from build123d import *

# Parameters (mm, degrees)
EXTRUDE_1_DEPTH       = 7
FILLET_1_R            = 10
CHAMFER_1_SIZE        = 5
CHAMFER_2_SIZE        = 2
SKETCH_3_R            = 4
CUT_EXTRUDE_2_DEPTH   = 98.811761039
SKETCH_5_W            = 7.308921848
SKETCH_5_H            = 35.296607786
CUT_EXTRUDE_2_2_DEPTH = 98.534926302


with BuildPart() as part:
    # Эскиз1 → Вытянуть1 (new body)
    with BuildSketch(Plane(origin=(0, 0, 0), x_dir=(0, 0, -1), z_dir=(1, 0, 0))):
        Polygon((62.822655934, -30.891323454), (59.120013374, -21.327683482), (30.956731402, -21.327683482), (30.956731402, -0.888409733), (92.539330922, -0.888409733), (92.539330922, -30.896809382), align=None)
    extrude(amount=-EXTRUDE_1_DEPTH)

    # Скругление1
    fillet_1_edges = [part.edges().sort_by_distance(p)[0] for p in [
        (-3.5, -21.327683482, -59.120013374),
    ]]
    fillet(fillet_1_edges, radius=FILLET_1_R)

    # Фаска1
    chamfer_1_edges = [part.edges().sort_by_distance(p)[0] for p in [
        (-3.5, -21.327683482, -30.956731402),
        (-3.5, -0.888409733, -30.956731402),
    ]]
    chamfer(chamfer_1_edges, length=CHAMFER_1_SIZE)

    # Фаска2
    chamfer_2_edges = [part.edges().sort_by_distance(p)[0] for p in [
        (0, -15.892609557, -92.539330922),
    ]]
    chamfer(chamfer_2_edges, length=CHAMFER_2_SIZE)

    # Эскиз3 → Cut-Extrude 2 (cut, through all)
    with BuildSketch(Plane.ZY.offset(7)):
        with Locations((-44.770273228, -12.131888622)):
            Circle(SKETCH_3_R)
    extrude(amount=-CUT_EXTRUDE_2_DEPTH, mode=Mode.SUBTRACT)

    # Эскиз5 → Cut-Extrude 2 2 (cut, through all)
    with BuildSketch(Plane(origin=(0, -30.879724855, 0.005700636), x_dir=(1, 0, 0), z_dir=(0, -0.9999999829599957, 0.0001846077143906597))):
        with Locations((-9.634460924, -46.111441198)):
            Rectangle(SKETCH_5_W, SKETCH_5_H)
    extrude(amount=-CUT_EXTRUDE_2_2_DEPTH, mode=Mode.SUBTRACT)


solid = part.part
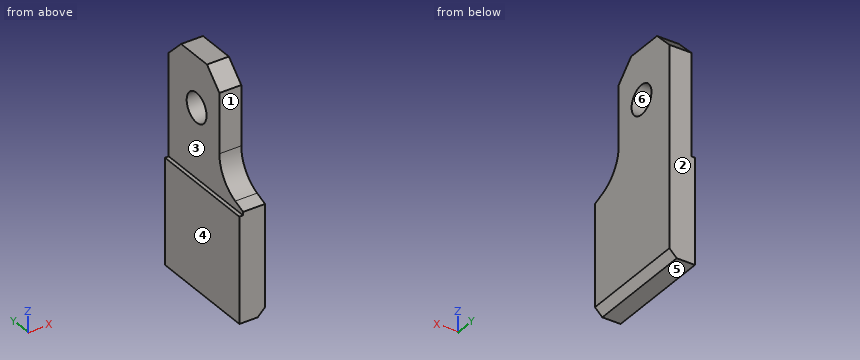
For this review, take the finished solid that the model builds, in its own axes (mm). Face numbers are marked on the shaded views. A direction names the side the tool comes from. Round coordinates to 2 decimals unless told otherwise and drop trailing zeros. Loops run counter-clockwise (first coordinate to the right, second up) from the corner with the lowest first, then second, coordinate; pieces in that order, holes last. Notation, with made-up numbers: (62, 86.5) - (94, 86.5) arc R20 ccw to (94, 94.5) - close; hole circle Ø5 at (63.25, 67.5). An arc over 180 degrees is marked (long way). Put each result on its own line as item: value. Start each with the question number.
1. For the marked faces 1, 2 and 3, list the 3-axis set-ups (+Z, -Z, +X, -X, +Y, -Y) from which the entire face can be reached by the end or side of a thin tool; tool diameter is ignored.
2. Consider section B-B on x = -1. State the section outline as (y, z) points, plus the area to 3 significant figures.
3. Consider section A-A on y = -13.5. State the section outline as (x, z) points, plus the area to 3 significant figures.
4. Consider section C-C on z = -43.5. State the section outline as (x, y) points.
5. Consider section D-D on y = -24.5. State the section outline as (x, z) points, plus the area to 3 significant figures.
6. For probe 1 along X at (y, z) = (-11, -35.5); probe 2 along Y at (x, z) = (-0.25, -80.5); probe 3 along Y at (x, z) = (-2, -40), list the stretches that pass through material, from the lowest coordinate up. Write a range as [from, to].
7. Insertion check: P1, Ø9, axis at y = -18.5, z = -51, coming from the -X side; P2, Ø0.8, axis at x = -6.5, y = -20.5, coming from the +Z side. Each pin has a flat end and moves straight along its axis. Give the tip position at first contact, or say it passes through.
8. Mouldability with a two-part tool opening along Z and no side actions: class the marked faces 4, 5 and 6 as +Z half, -Z half, draft (parallel to the pull), parting line (faces both ways), or undercut.
Result sheet:
1. face 1: +Z, +X, -X, -Y
1. face 2: +Z, -Z, +X, -X, +Y
1. face 3: +Z, -X, +Y, -Y
2. outline: (-30.9, -91.54) - (-0.89, -91.54) - (-0.89, -35.96) - (-5.89, -30.96) - (-16.33, -30.96) - (-21.33, -35.96) - (-21.33, -52.27) arc R10 cw to (-27.72, -61.59) - (-30.89, -62.82) - close; hole circle Ø8 at (-12.13, -44.77)
2. area: 1,460 mm^2
3. outline: (-7, -92.54) - (-2, -92.54) - (0, -90.54) - (0, -48.53) - (-5.98, -48.53) - (-5.98, -63.76) - (-7, -63.76) - close; (-5.98, -41.01) - (0, -41.01) - (0, -30.96) - (-5.98, -30.96) - close
3. area: 351 mm^2
4. outline: (-5.98, -21.33) - (0, -21.33) - (0, -15.92) - (-5.98, -15.92) - close; (-5.98, -8.34) - (0, -8.34) - (0, -0.89) - (-5.98, -0.89) - close
5. outline: (-7, -92.54) - (-2, -92.54) - (0, -90.54) - (0, -59.57) - (-5.98, -59.57) - (-5.98, -63.76) - (-7, -63.76) - close
5. area: 224 mm^2
6. probe 1: [-5.98, 0]
6. probe 2: [-30.89, -0.89]
6. probe 3: [-21.33, -0.89]
7. P1: x = -5.98
7. P2: z = -63.76
8. face 4: draft
8. face 5: -Z half
8. face 6: undercut
